Here's how the part is built. I have some questions about the finished solid (model axes, mm). A direction names the side the tool comes from. Coordinates: 2 decimals unless noted, no trailing zeros. Order: outer loops, then holes, each group sorted by start corner. A loop starts at its lowest first (then second) coordinate and runs counter-clockwise, first axis right, second up. Notation, with made-up numbers: (-28, -11.5) - (-24, -11.5) arc R21 ccw to (-24, -3.5) - close; hole circle Ø5 at (-22.75, 33). An arc over 180 degrees is marked (long way). Answer in a Markdown table with one row per item. Add a question column.
Item 1: On a 3-axis mill with a long thin cutter (end or side, diameter ignored), from which of +Z, -Z, +X, -X, +Y, -Y can I reach the whole of each face in a straight line? I mean faces 1 (the flat face through (-4, -2.54, -5.5)), 2 (the flat face through (-4, -3, -6.01)), 3 (the flat face through (2.723, -3, 0)), 4 (the flat face through (3, -2.54, -6)), 5 (the flat face through (5.3, -2.54, -1.3)). Say none if no direction works.
Item 2: I want a section at D-D (x = -3.5). Please give me the cut outline in (y, z).
Item 3: I want a section at A-A (y = -3.6). Please give me the cut outline in (x, z).
Item 4: If I drill on line 1 along Z through (x, y) = (0, -1.35); line 2 along X through (y, z) = (-2.9, 0.75); line 3 along X through (y, z) = (-3.6, -2), over which ranges is the centre line in solid material (lowest first)? Write a range as from..to.
Item 5: Will these pins go through, and if not, where does the flat tip stop? pin 1 Ø1.8 at (x, z) = (-4, 5.5) entering from +Y; pin 2 Ø1.4 at (y, z) = (-3.5, -2) entering from +X; pin 3 Ø1 at (x, z) = (-5.5, -0.5) entering from -Y; pin 4 Ø1.4 at (x, y) = (-4, -3) entering from +Z.
Item 6: I want a section at B-B (x = 0). Please give me the cut outline in (y, z).
Item 7: Thinking about a two-plate mould opening in X: for faces 6 (the cylindrical face through (2.93, -0.97, -5.634)), 7 (the flat face through (-5, -2.54, 0)), 8 (the flat face through (0, -3, -0.801)), 9 (the flat face through (-4.647, -3, 0)), which applies, +X half, -X half, draft (parallel to the pull), parting line (faces both ways), or undercut?
```python
from build123d import *

# Parameters (mm, degrees)
F0_R          = 6.35
F1_DEPTH      = 2.54
F2_W          = 1.6741803847
F2_H          = 6.0100271367
F3_DEPTH      = 1.27
F4_W          = 5.4453448392
F4_H          = 0.8010258316
F5_DEPTH      = 1.27
F7_DEPTH      = 1.27
F8_R          = 0.7810995879
F9_DEPTH      = 25.4
F10_T4_ANGLE  = 60.776700367
F10_T9_ANGLE  = 70.6868696842
F10_T15_ANGLE = 108.8474457798
F10_T20_ANGLE = 95.5948420913
F10_T26_ANGLE = 35.8710937336


# Not quite as in the source:
# - a fillet or chamfer that OpenCascade refuses, or shapes differently, is made with other operations: its cross-section is extruded or revolved along the edge and cut away or added
# - a feature of the source that left no trace in its solid (it failed there, or was rolled back) is left out


with BuildPart() as f1:
    # F0 (on Front) → F1 (new body)
    with BuildSketch(Plane.XZ):
        Circle(F0_R)
    extrude(amount=F1_DEPTH)

    # F2 (on face) → F3 (join)
    with BuildSketch(Plane.XZ.offset(2.54)):
        with Locations((-3.81, 3.0050135683)):
            Rectangle(F2_W, F2_H)
        with Locations((-3.81, -3.0050135683)):
            Rectangle(F2_W, F2_H)
    extrude(amount=F3_DEPTH)

    # F4 (on face) → F5 (join)
    with BuildSketch(Plane.XZ.offset(2.54)):
        with Locations((0, 0.4005129158)):
            Rectangle(F4_W, F4_H)
        with Locations((0, -0.4005129158)):
            Rectangle(F4_W, F4_H)
    extrude(amount=F5_DEPTH)

    # F6 (on face) → F7 (join)
    with BuildSketch(Plane.XZ.offset(2.54)):
        Polygon((4.6705882996, 5.4137986153), (2.1562074386, -5.9727103966), (1.9563709538, -6.8768215956), (3.6039068937, -7.2406322096), (6.3179433579, 5.0500279438), align=None)
    extrude(amount=F7_DEPTH)

    # F8 (on face) → F9 (cut)
    with BuildSketch(Plane.XZ.offset(2.54)):
        with Locations((0, 5.1177083515)):
            Circle(F8_R)
    extrude(amount=-F9_DEPTH, mode=Mode.SUBTRACT)

    # F10: fillet of radius 0.508 on 5 edges, made by hand


with BuildPart() as f10_tool2:
    # F10_s3 → F10_t4 (revolve)
    with BuildSketch(Plane(origin=(0, 0, 0), x_dir=(0, 1, 0), z_dir=(-0.8727236144, 0, -0.4882145972))):
        with BuildLine():
            ThreePointArc((-2.032, 6.35), (-2.3912102448, 6.2012102448), (-2.54, 5.842))
            Line((-2.54, 5.842), (-2.54, 6.35))
            Line((-2.54, 6.35), (-2.032, 6.35))
        make_face()
    revolve(axis=Axis((0, -2.54, 0), (0, -1, 0)), revolution_arc=F10_T4_ANGLE)

    split(bisect_by=Plane(origin=(4.9608883724, 0, -1.0954685729), x_dir=(0, 1, 0), z_dir=(0.9764759285, 0, -0.2156264386)), keep=Keep.TOP)


with BuildPart() as f1_1:
    add(f1.part)

    # F10_t1: cut F10_tool2
    add(f10_tool2.part, mode=Mode.SUBTRACT)


with BuildPart() as f10_tool7:
    # F10_s8 → F10_t9 (revolve)
    with BuildSketch(Plane(origin=(0, 0, 0), x_dir=(0, 1, 0), z_dir=(-0.7729956778, 0, 0.6344112878))):
        with BuildLine():
            ThreePointArc((-2.032, 6.35), (-2.3912102448, 6.2012102448), (-2.54, 5.842))
            Line((-2.54, 5.842), (-2.54, 6.35))
            Line((-2.54, 6.35), (-2.032, 6.35))
        make_face()
    revolve(axis=Axis((0, -2.54, 0), (0, -1, 0)), revolution_arc=F10_T9_ANGLE)

    split(bisect_by=Plane.YZ.offset(-2.9729098076), keep=Keep.TOP)

    split(bisect_by=Plane(origin=(3.313533314, 0, -0.7316979013), x_dir=(0, 1, 0), z_dir=(-0.9764759285, 0, 0.2156264386)), keep=Keep.TOP)


with BuildPart() as f1_2:
    add(f1_1.part)

    # F10_t6: cut F10_tool7
    add(f10_tool7.part, mode=Mode.SUBTRACT)


with BuildPart() as f10_tool13:
    # F10_s14 → F10_t15 (revolve)
    with BuildSketch(Plane(origin=(0, 0, 0), x_dir=(0, 1, 0), z_dir=(0.813341715, 0, 0.581786262))):
        with BuildLine():
            ThreePointArc((-2.032, 6.35), (-2.3912102448, 6.2012102448), (-2.54, 5.842))
            Line((-2.54, 5.842), (-2.54, 6.35))
            Line((-2.54, 6.35), (-2.032, 6.35))
        make_face()
    revolve(axis=Axis((0, -2.54, 0), (0, -1, 0)), revolution_arc=F10_T15_ANGLE)

    split(bisect_by=Plane.YZ.offset(-4.6470901924), keep=Keep.BOTTOM)


with BuildPart() as f1_3:
    add(f1_2.part)

    # F10_t12: cut F10_tool13
    add(f10_tool13.part, mode=Mode.SUBTRACT)


with BuildPart() as f10_tool18:
    # F10_s19 → F10_t20 (revolve)
    with BuildSketch(Plane(origin=(0, 0, 0), x_dir=(0, 1, 0), z_dir=(0.5560518892, 0, -0.8311475781))):
        with BuildLine():
            ThreePointArc((-2.032, 6.35), (-2.3912102448, 6.2012102448), (-2.54, 5.842))
            Line((-2.54, 5.842), (-2.54, 6.35))
            Line((-2.54, 6.35), (-2.032, 6.35))
        make_face()
    revolve(axis=Axis((0, -2.54, 0), (0, -1, 0)), revolution_arc=F10_T20_ANGLE)

    split(bisect_by=Plane.YZ.offset(-2.9729098076), keep=Keep.TOP)

    split(bisect_by=Plane(origin=(3.313533314, 0, -0.7316979013), x_dir=(0, 1, 0), z_dir=(-0.9764759285, 0, 0.2156264386)), keep=Keep.TOP)


with BuildPart() as f1_4:
    add(f1_3.part)

    # F10_t17: cut F10_tool18
    add(f10_tool18.part, mode=Mode.SUBTRACT)


with BuildPart() as f10_tool24:
    # F10_s25 → F10_t26 (revolve)
    with BuildSketch(Plane.XY):
        with BuildLine():
            ThreePointArc((6.35, -2.032), (6.2012102448, -2.3912102448), (5.842, -2.54))
            Line((5.842, -2.54), (6.35, -2.54))
            Line((6.35, -2.54), (6.35, -2.032))
        make_face()
    revolve(axis=Axis((0, -2.54, 0), (0, -1, 0)), revolution_arc=F10_T26_ANGLE)

    split(bisect_by=Plane(origin=(4.9608883724, 0, -1.0954685729), x_dir=(0, 1, 0), z_dir=(0.9764759285, 0, -0.2156264386)), keep=Keep.TOP)


with BuildPart() as f1_5:
    add(f1_4.part)

    # F10_t23: cut F10_tool24
    add(f10_tool24.part, mode=Mode.SUBTRACT)


solid = f1_5.part
```
Values follow:
| question | item | result |
|---|---|---|
| 1 | face 1 | -Z, -X, +Y |
| 1 | face 2 | -Z, -X, +Y, -Y |
| 1 | face 3 | +Z, -Y |
| 1 | face 4 | -Z, +X, +Y |
| 1 | face 5 | -Z, +X, -Y |
| 2 | outline | (-3.81, -6.01) - (-2.54, -6.01) - (-2.54, -5.3) - (0, -5.3) - (0, 5.3) - (-2.54, 5.3) - (-2.54, 6.01) - (-3.81, 6.01) - close |
| 3 | outline | (-4.65, -6.01) - (-2.97, -6.01) - (-2.97, 6.01) - (-4.65, 6.01) - close; (-2.72, -0.8) - (2.72, -0.8) - (2.72, 0.8) - (-2.72, 0.8) - close; (1.96, -6.88) - (3.6, -7.24) - (6.32, 5.05) - (4.67, 5.41) - (2.16, -5.97) - close |
| 4 | line 1 | z = -6.35..4.34, 5.9..6.35 |
| 4 | line 2 | x = -4.65..-2.97, -2.72..2.72, 3.64..5.37 |
| 4 | line 3 | x = -4.65..-2.97, 3.03..4.76 |
| 5 | pin 1 | stops at y = 0 |
| 5 | pin 2 | stops at x = 4.92 |
| 5 | pin 3 | stops at y = -2.54 |
| 5 | pin 4 | stops at z = 6.01 |
| 6 | outline | (-3.81, -0.8) - (-2.54, -0.8) - (-2.54, -5.84) arc R0.51 ccw to (-2.03, -6.35) - (0, -6.35) - (0, 4.34) - (-2.54, 4.34) - (-2.54, 0.8) - (-3.81, 0.8) - close; (-2.54, 5.9) - (0, 5.9) - (0, 6.35) - (-2.03, 6.35) arc R0.51 ccw to start |
| 7 | face 6 | parting line |
| 7 | face 7 | draft |
| 7 | face 8 | undercut |
| 7 | face 9 | -X half |
